Source: three-view drawing plus pictorial views. Frame: mm from the lowest corner of the part. A direction names the side the tool comes from. Give positions to 0.01 mm unless a question says otherwise; leave off trailing zeros. Order: outer loops, then holes, each group sorted by start corner. A loop starts at its lowest first (then second) coordinate and runs counter-clockwise, first axis right, second up.
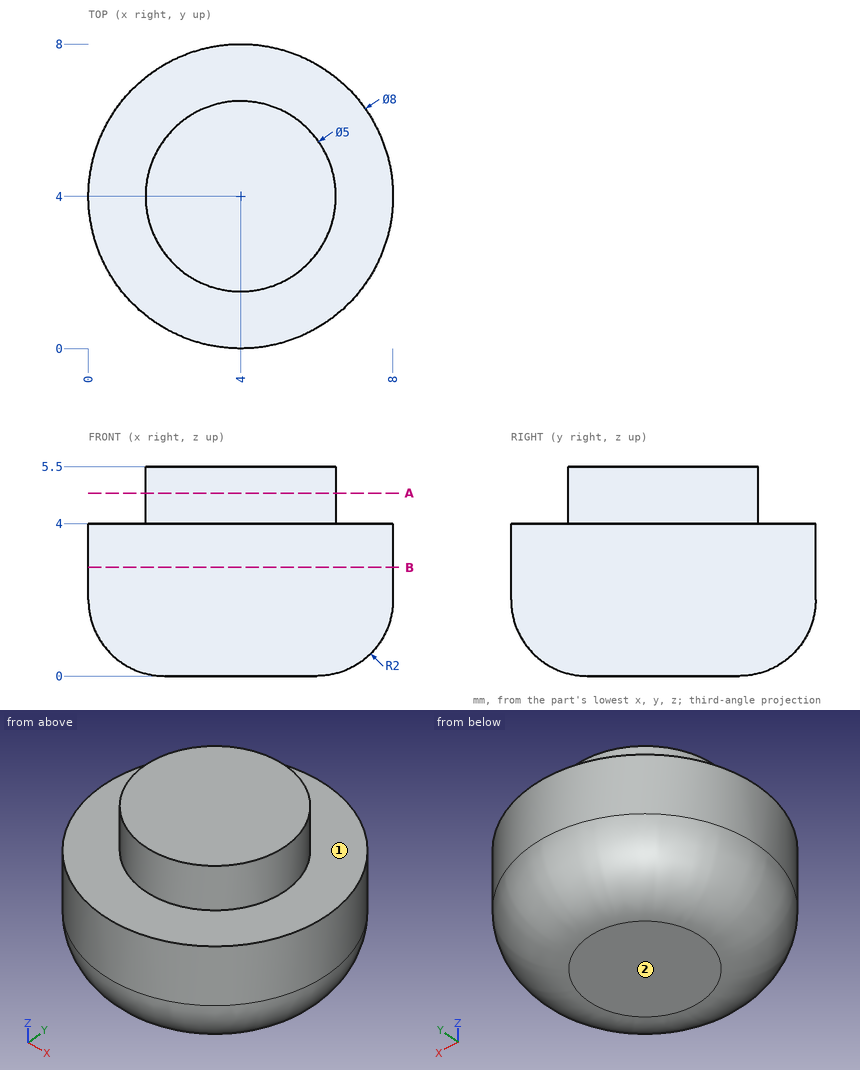
1) Ray query, L1, parallel to X at y = 2.5, z = 4.65; L2, parallel to X at y = 7.5, z = 2.1; L3, parallel to Y at x = 3.75, z = 2.4. Return the intervals inside material, ascending.
Checks:
L1: x = 2 to 6
L2: x = 2.06 to 5.94
L3: y = 0.01 to 7.99
2) Section query B-B on z = 2.85. Output: boundary loops of the cut face in (x, y), and give its area (3 significant figures).
Checks:
outline: circle Ø8 at (4, 4)
area: 50.3 mm2
3) Reachability of the marked faces 1 and 2 from +Z, -Z, +X, -X, +Y, -Y: full face, straight path, thin tool, end or side. Return the list, or none.
Checks:
face 1: +Z
face 2: -Z, +X, -X, +Y, -Y
4) Section query A-A on z = 4.8. Output: boundary loops of the cut face in (x, y).
Checks:
outline: circle Ø5 at (4, 4)
